from build123d import *

# Parameters (mm, degrees)
BOSS_EXTRUDE1_DEPTH = 3


with BuildPart() as part:
    # Model → Boss-Extrude1 (new body)
    with BuildSketch(Plane.XY):
        with BuildLine():
            Line((1130.2, -228.052661621), (1130.2, -248.052661621))
            Line((1130.2, -248.052661621), (1160.2, -248.052661621))
            Line((1160.2, -248.052661621), (1160.2, -200.422661621))
            Line((1160.2, -200.422661621), (1207.901037796, -200.422661621))
            Line((1207.901037796, -200.422661621), (1207.901037796, -245.979700014))
            Line((1207.901037796, -245.979700014), (1210.901037796, -245.979700014))
            Line((1210.901037796, -245.979700014), (1210.901037796, -200.422661621))
            Line((1210.901037796, -200.422661621), (1366.901037796, -200.422661621))
            Line((1366.901037796, -200.422661621), (1366.901037796, -245.979700014))
            Line((1366.901037796, -245.979700014), (1369.901037796, -245.979700014))
            Line((1369.901037796, -245.979700014), (1369.901037796, -200.422661621))
            Line((1369.901037796, -200.422661621), (1525.901037796, -200.422661621))
            Line((1525.901037796, -200.422661621), (1525.901037796, -245.979700014))
            Line((1525.901037796, -245.979700014), (1528.901037796, -245.979700014))
            Line((1528.901037796, -245.979700014), (1528.901037796, -200.422661621))
            Line((1528.901037796, -200.422661621), (1684.901037801, -200.422661621))
            Line((1684.901037801, -200.422661621), (1684.901037801, -245.979700014))
            Line((1684.901037801, -245.979700014), (1687.901037795, -245.979700014))
            Line((1687.901037795, -245.979700014), (1687.901037795, -200.422661621))
            Line((1687.901037795, -200.422661621), (1756.943542984, -200.422661621))
            Line((1756.943542984, -200.422661621), (1756.943542984, -245.979700014))
            Line((1756.943542984, -245.979700014), (1759.943542984, -245.979700014))
            Line((1759.943542984, -245.979700014), (1759.943542984, -200.422661621))
            Line((1759.943542984, -200.422661621), (1828.986048173, -200.422661621))
            Line((1828.986048173, -200.422661621), (1828.986048173, -245.979700014))
            Line((1828.986048173, -245.979700014), (1831.986048173, -245.979700014))
            Line((1831.986048173, -245.979700014), (1831.986048173, -200.422661621))
            Line((1831.986048173, -200.422661621), (1901.028553362, -200.422661621))
            Line((1901.028553362, -200.422661621), (1901.028553362, -245.979700014))
            Line((1901.028553362, -245.979700014), (1904.028553362, -245.979700014))
            Line((1904.028553362, -245.979700014), (1904.028553362, -200.422661621))
            Line((1904.028553362, -200.422661621), (1973.071058551, -200.422661621))
            Line((1973.071058551, -200.422661621), (1973.071058551, -245.979700014))
            Line((1973.071058551, -245.979700014), (1976.071058551, -245.979700014))
            Line((1976.071058551, -245.979700014), (1976.071058551, -200.422661621))
            Line((1976.071058551, -200.422661621), (2045.113563739, -200.422661621))
            Line((2045.113563739, -200.422661621), (2045.113563739, -245.979700014))
            Line((2045.113563739, -245.979700014), (2048.11356374, -245.979700014))
            Line((2048.11356374, -245.979700014), (2048.11356374, -267.236738408))
            add(Edge.make_bspline(
                [(2048.11356374, -267.236738408), (1921.116123258, -299.875981212), (1758.376470444, -319.638055471), (1545.730966639, -313)],
                knots=[0.571508356, 0.571508356, 0.571508356, 0.571508356, 1, 1, 1, 1], degree=3))
            add(Edge.make_bspline(
                [(1545.730966639, -313), (1417.219843878, -313.786784413), (1288.709572371, -314.686711241), (1160.2, -315.679561973)],
                knots=[0, 0, 0, 0, 1, 1, 1, 1], degree=3))
            Line((1160.2, -315.679561973), (1160.2, -268.052661621))
            Line((1160.2, -268.052661621), (1130.2, -268.052661621))
            Line((1130.2, -268.052661621), (1130.2, -288.052661621))
            ThreePointArc((1130.2, -288.052661621), (1100.2, -258.052661621), (1130.2, -228.052661621))
        make_face()
    extrude(amount=BOSS_EXTRUDE1_DEPTH)


solid = part.part
Work out the finished part from the listing and answer in its coordinate system (mm). Round coordinates to 2 decimals unless told otherwise and drop trailing zeros. Write each question's results on one line, items separated by ' | '.
Item 1: Find the intervals of material crossed by line 1 along Y through (x, z) = (1641.5, 2.4); line 2 along Y through (x, z) = (1665, 2.5); line 3 along X through (y, z) = (-251, 2), in increasing order. Write a range as [from, to].
Result set:
line 1: [-314.23, -200.42] | line 2: [-313.96, -200.42] | line 3: [1101.04, 2048.11]
Item 2: A cutting plane is placed at A-A, the plane y = -236. Count the separate pieces of the cut face and the enclosed holes in it, plus the area to 3 significant figures.
Result set:
separate pieces: 10 | enclosed holes: 0 | area: 2,640 mm^2
Item 3: Flat-ended cylindrical pins translate along their axes: P1, Ø1.5, axis at x = 1975, z = 1, coming from the +Y side; P2, Ø1, axis at y = -247, z = 2.5, coming from the -X side. Find the tip coordinate at first contact, or state that the pin passes through.
Result set:
P1: y = -245.98 | P2: x = 1102.12
